Input: dimensioned drawing with shaded views. Units: mm. Origin: part minimum x, y, z. Round coordinates to 2 decimals unless told otherwise and drop trailing zeros. Order: outer loops, then holes, each group sorted by start corner. A loop starts at its lowest first (then second) coordinate and runs counter-clockwise, first axis right, second up. Notation, with made-up numbers: M -24,31.5 L 25,31.5 A21 cw 25,70.5 Z; hole C 8,-25 d3. An arc over 180 degrees is marked long. Put each result on its own line as item: value. Start each with the question number.
1) Section C-C, the plane x = 4. Return loops of the section in (y, z) (1 decimal).
2) Section A-A, the plane x = 15.75. Return loops of the section in (y, z) (1 decimal).
3) Section D-D, the plane y = 8.25. Return loops of the section in (x, z).
4) Material intervals for probe 1 along Y at (x, z) = (27.75, 0.85) (1 decimal); probe 2 along Y at (x, z) = (20, 0.55) (1 decimal); probe 3 along X at (y, z) = (6, 0.8) (1 decimal), sorted ascending. Write a range as [from, to].
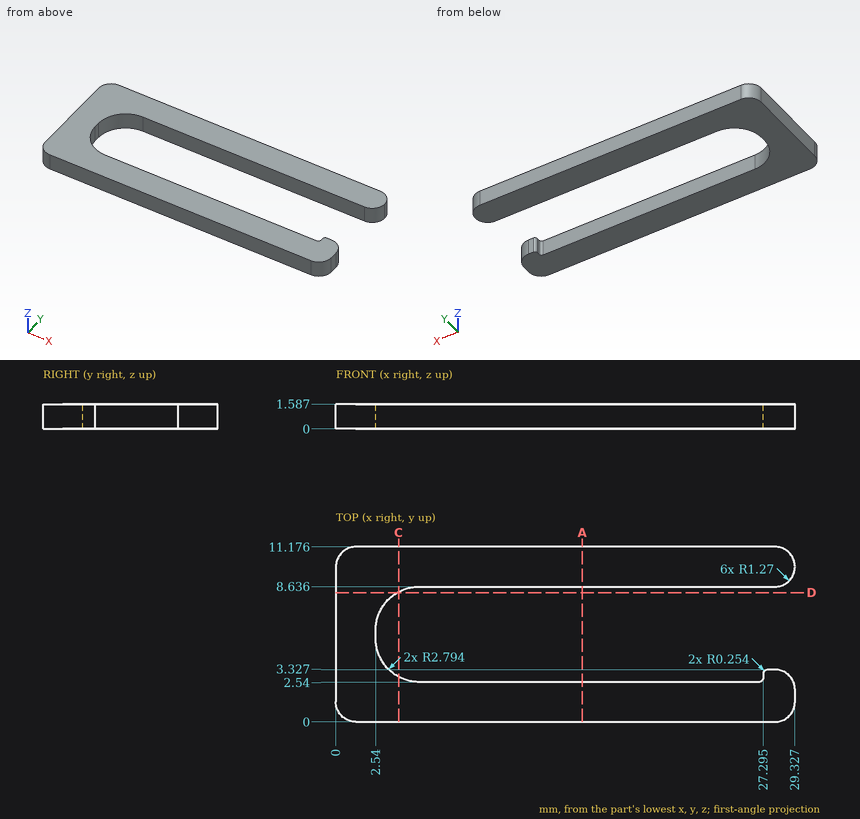
Result sheet:
1. outline: M 0,0 L 2.9,0 L 2.9,1.6 L 0,1.6 Z; M 8.3,0 L 11.2,0 L 11.2,1.6 L 8.3,1.6 Z
2. outline: M 0,0 L 2.5,0 L 2.5,1.6 L 0,1.6 Z; M 8.6,0 L 11.2,0 L 11.2,1.6 L 8.6,1.6 Z
3. outline: M 0,0 L 3.92,0 L 3.92,1.59 L 0,1.59 Z
4. probe 1: y = [0, 3.3], [8.6, 11.2]
4. probe 2: y = [0, 2.5], [8.6, 11.2]
4. probe 3: x = [0, 2.5]
